Autodesk Inventor part; units mm, degrees
ref_plane "YZ Plane" through (0, 0, 0) normal (1, 0, 0) x (0, 1, 0)
ref_plane "XZ Plane" through (0, 0, 0) normal (0, 1, 0) x (-1, 0, 0)
ref_plane "XY Plane" through (0, 0, 0) normal (0, 0, 1) x (1, 0, 0)
sketch "Sketch1" plane through (0, 0, 0) normal (0, 0, 1) x (1, 0, 0)
  line L0 (-11.5, -75) -> (11.5, -75)
  line L1 (11.5, -75) -> (11.5, 75)
  line L2 (11.5, 75) -> (-11.5, 75)
  line L3 (-11.5, 75) -> (-11.5, -75)
  line L4 (-11.5, -75) -> (11.5, 75) construction
  line L5 (11.5, -75) -> (-11.5, 75) construction
  line L6 (-4.5, 75) -> (4.5, 75)
  line L7 (4.5, 75) -> (4.5, -5)
  line L8 (4.5, -5) -> (-4.5, -5) construction
  line L9 (-4.5, -5) -> (-4.5, 75)
  line L10 (0, -75) -> (0, 75) construction
  line L11 (-4.5, -5) -> (-11.5, -5)
  line L12 (4.5, -5) -> (11.5, -5)
  point P0 (0, 0)
  dimension "d0" = 150
  dimension "d1" = 80
  dimension "d2" = 7
  dimension "d3" = 23
extrude "Extrusion1" add sketch "Sketch1" against normal blind 20 contours L3 L11 L9 L2 L7 L12 L1 L0
chamfer "Chamfer1" distance 2 angle 45 7 edges at (0, -75, 0) (-11.5, -40, 0) (11.5, -40, 0) (8, -5, 0) (-8, -5, 0) (-4.5, 35, 0) (4.5, 35, 0)
equation "\"d0\" = key_length"
equation "\"d1\" = blackkey_length"
equation "\"d2\" = blackkey_halfwidth"
equation "\"d3\" = key_width"
equation "\"d4\" = key_height"
properties part number "key_3"
Build history of the part. All positions in model axes, mm. A direction names the side the tool comes from. Round coordinates to 2 decimals unless told otherwise and drop trailing zeros. Write each loop counter-clockwise with the first axis right and the second up, starting at its lowest first coordinate (ties: lowest second). Pieces come first, ordered by that corner, then holes. Notation, with made-up numbers: M 22.5,-10.75 L 56.5,-10.75 A21 cw 56.5,-1.75 Z; hole C 3,35 d8. An arc over 180 degrees is marked long. Answer as a JSON object with one key per item and string values. Group by question number.
(1) Flat gauge pins, fed straight in: pin 1 (1.5 mm diameter, centred on y = 3.5, z = -3, fed in from -X); pin 2 (2 mm diameter, centred on x = -9.5, z = -14, fed in from +Y); pin 3 (4 mm diameter, centred on x = -9, y = -4.5, fed in from +Z). Where does each tip first touch, or does it go through?
(2) Cut at B-B (z = -18.5). Give the cut face in (x, y).
(3) Which spindle directions (+Z, -Z, +X, -X, +Y, -Y) get a long thin tool onto all of the face, cutting with end or side? Do faces 1 (the flat face through (4.5, 36, -11)), 2 (the flat face through (-8, -5, -11)), 3 (the flat face through (0, -14, 0)). Say none if no direction does.
(4) Cut at A-A (y = 18). Give the cut face in (x, z).
(5) Cut at C-C (x = -6). Give the cut face in (y, z).
(6) Drill centre lines: L1, parallel to X at y = 51.5, z = -7.75; L2, parallel to Y at x = -6, z = -14.25; L3, parallel to Z at x = 2.75, y = 15. Where is each one in solid material? Low to high.
Responses:
{
 "1": {"pin 1": "stops at x = -4.5", "pin 2": "stops at y = -5", "pin 3": "stops at z = -0.5"},
 "2": {"outline": "M -11.5,-75 L 11.5,-75 L 11.5,-5 L 4.5,-5 L 4.5,75 L -4.5,75 L -4.5,-5 L -11.5,-5 Z"},
 "3": {"face 1": "+Z, -Z, +X, +Y", "face 2": "+Z, -Z, -X, +Y", "face 3": "+Z, +X, -X, +Y, -Y"},
 "4": {"outline": "M -4.5,-20 L 4.5,-20 L 4.5,-2 L 2.5,0 L -2.5,0 L -4.5,-2 Z"},
 "5": {"outline": "M -75,-20 L -5,-20 L -5,-2 L -7,0 L -73,0 L -75,-2 Z"},
 "6": {"L1": "x = -4.5 to 4.5", "L2": "y = -75 to -5", "L3": "z = -20 to -0.25"}
}
